The model under review builds one solid part; all positions refer to its coordinate system, in mm. Face numbers are marked on the shaded views. A direction names the side the tool comes from. Give positions to 0.01 mm unless a question says otherwise; leave off trailing zeros. Write each loop counter-clockwise with the first axis right and the second up, starting at its lowest first coordinate (ties: lowest second). Pieces come first, ordered by that corner, then holes. Notation, with made-up numbers: (9.5, 64) -> (44.5, 64) arc R4 ccw to (44.5, 71) -> close; hole circle Ø7 at (-1.5, -3.75). An arc over 180 degrees is marked (long way). Use CSV: the item, a comma, the result in double quotes.
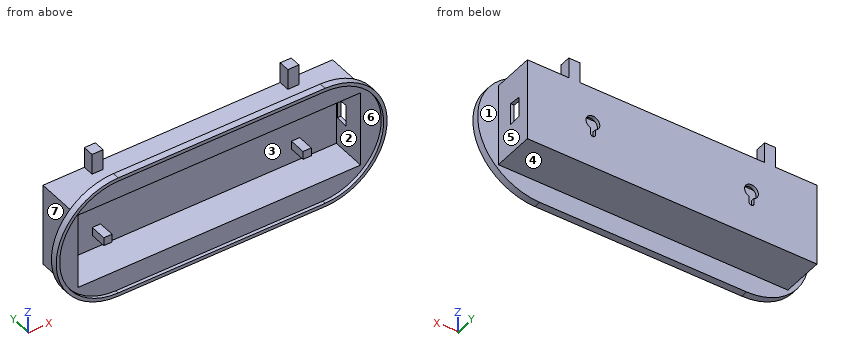
```python
from build123d import *

# Parameters (mm, degrees)
F0_W      = 266.7
F0_H      = 76.2
F1_DEPTH  = 3.175
F2_W      = 266.7
F2_H      = 76.2
F2_W_2    = 260.35
F2_H_2    = 69.85
F3_DEPTH  = 28.956
F4_W      = 260.35
F4_H      = 69.85
F5_DEPTH  = 6.35
F7_DEPTH  = 3.175
F8_W      = 266.7
F8_H      = 76.2
F8_W_2    = 19.05
F8_H_2    = 25.4
F9_DEPTH  = 6.35
F10_W     = 19.05
F10_H     = 25.4
F11_DEPTH = 3.175
F13_DEPTH = 3.175
F14_W     = 10.16
F14_H     = 10.16
F15_DEPTH = 19.05
F16_W     = 7.62
F16_H     = 7.62
F17_DEPTH = 15.24


with BuildPart() as f1:
    # F0 (on Front) → F1 (new body)
    with BuildSketch(Plane.XZ):
        with Locations((133.35, -38.1)):
            Rectangle(F0_W, F0_H)
    extrude(amount=F1_DEPTH)

    # F2 (on face) → F3 (join)
    with BuildSketch(Plane.XZ.offset(3.175)):
        with Locations((133.35, -38.1)):
            Rectangle(F2_W, F2_H)
        with Locations((133.35, -38.1)):
            Rectangle(F2_W_2, F2_H_2, mode=Mode.SUBTRACT)
    extrude(amount=F3_DEPTH)

    # F4 (on face) → F5 (join)
    with BuildSketch(Plane.XZ.offset(32.131)):
        with BuildLine():
            Line((228.6, 19.05), (38.1, 19.05))
            ThreePointArc((38.1, 19.05), (-19.05, -38.1), (38.1, -95.25))
            Line((38.1, -95.25), (228.6, -95.25))
            ThreePointArc((228.6, -95.25), (285.75, -38.1), (228.6, 19.05))
        make_face()
        with Locations((133.35, -38.1)):
            Rectangle(F4_W, F4_H, mode=Mode.SUBTRACT)
    extrude(amount=F5_DEPTH)

    # F6 (on face) → F7 (cut)
    with BuildSketch(Plane.XZ.offset(38.481)):
        with BuildLine():
            Line((228.6, 15.875), (38.1, 15.875))
            ThreePointArc((38.1, 15.875), (-15.875, -38.1), (38.1, -92.075))
            Line((38.1, -92.075), (228.6, -92.075))
            ThreePointArc((228.6, -92.075), (282.575, -38.1), (228.6, 15.875))
        make_face()
    extrude(amount=-F7_DEPTH, mode=Mode.SUBTRACT)

    # F8 (on face) → F9 (join)
    with BuildSketch(Plane(origin=(0, 0, 0), x_dir=(-1, 0, 0), z_dir=(0, 1, 0))):
        with Locations((-133.35, -38.1)):
            Rectangle(F8_W, F8_H)
        with Locations((-206.375, -38.1)):
            Rectangle(F8_W_2, F8_H_2, mode=Mode.SUBTRACT)
        with Locations((-60.325, -38.1)):
            Rectangle(F8_W_2, F8_H_2, mode=Mode.SUBTRACT)
    extrude(amount=F9_DEPTH)

    # F10 (on face) → F11 (join)
    with BuildSketch(Plane(origin=(0, 6.35, 0), x_dir=(-1, 0, 0), z_dir=(0, 1, 0))):
        with Locations((-60.325, -38.1)):
            Rectangle(F10_W, F10_H)
        with BuildLine():
            ThreePointArc((-62.611, -39.198247), (-60.325, -26.924), (-58.039, -39.198247))
            Line((-58.039, -39.198247), (-58.039, -44.45))
            ThreePointArc((-58.039, -44.45), (-60.325, -46.736), (-62.611, -44.45))
            Line((-62.611, -44.45), (-62.611, -39.198247))
        make_face(mode=Mode.SUBTRACT)
        with Locations((-206.375, -38.1)):
            Rectangle(F10_W, F10_H)
        with BuildLine():
            ThreePointArc((-208.661, -39.198247), (-206.375, -26.924), (-204.089, -39.198247))
            Line((-204.089, -39.198247), (-204.089, -44.45))
            ThreePointArc((-204.089, -44.45), (-206.375, -46.736), (-208.661, -44.45))
            Line((-208.661, -44.45), (-208.661, -39.198247))
        make_face(mode=Mode.SUBTRACT)
    extrude(amount=-F11_DEPTH)

    # F12 (on face) → F13 (cut, through all)
    with BuildSketch(Plane.YZ.offset(266.7)):
        Polygon((-4.699, -47.3075), (-4.699, -28.8925), (-15.875, -27.94), (-15.875, -48.26), align=None)
    extrude(amount=-F13_DEPTH, mode=Mode.SUBTRACT)

    # F14 (on face) → F15 (join, through all)
    with BuildSketch(Plane.XY):
        with Locations((43.18, 1.27)):
            Rectangle(F14_W, F14_H)
        with Locations((223.52, 1.27)):
            Rectangle(F14_W, F14_H)
    extrude(amount=F15_DEPTH)

    # F16 (on face) → F17 (join)
    with BuildSketch(Plane.XZ.offset(3.175)):
        with Locations((226.0092, -56.007)):
            Rectangle(F16_W, F16_H)
        with Locations((226.0092, -13.843)):
            Rectangle(F16_W, F16_H)
        with Locations((42.545, -56.007)):
            Rectangle(F16_W, F16_H)
        with Locations((42.545, -13.843)):
            Rectangle(F16_W, F16_H)
    extrude(amount=F17_DEPTH)


solid = f1.part
```
Q1. Consider section C-C (x = 123). Write out the cut boundary in (y, z) (3 decimals), then the cut area to 3 significant figures.
Derived:
outline,"(-38.481, -95.25) -> (-32.131, -95.25) -> (-32.131, -76.2) -> (6.35, -76.2) -> (6.35, 0) -> (-32.131, 0) -> (-32.131, 19.05) -> (-38.481, 19.05) -> (-38.481, 15.875) -> (-35.306, 15.875) -> (-35.306, -3.175) -> (-3.175, -3.175) -> (-3.175, -73.025) -> (-35.306, -73.025) -> (-35.306, -92.075) -> (-38.481, -92.075) -> close"
area,"1,070 mm2"
Q2. Consider section B-B (z = 12). Write out the cut boundary in (x, y), then the cut area to 3 significant figures.
Derived:
outline,"(10.6, -38.48) -> (18.02, -38.48) -> (18.02, -35.31) -> (248.68, -35.31) -> (248.68, -38.48) -> (256.1, -38.48) -> (256.1, -32.13) -> (10.6, -32.13) -> close; (38.1, -3.81) -> (48.26, -3.81) -> (48.26, 6.35) -> (38.1, 6.35) -> close; (218.44, -3.81) -> (228.6, -3.81) -> (228.6, 6.35) -> (218.44, 6.35) -> close"
area,"1,030 mm2"
Q3. Consider section D-D (z = -81.5). Write out the cut boundary in (x, y), then the cut area to 3 significant figures.
Derived:
outline,"(0.92, -38.48) -> (6.01, -38.48) -> (6.01, -35.31) -> (260.69, -35.31) -> (260.69, -38.48) -> (265.78, -38.48) -> (265.78, -32.13) -> (0.92, -32.13) -> close"
area,"873 mm2"
Q4. Machinability: for the marked faces 5, 6 and 7, which of the approach directions +Z, -Z, +X, -X, +Y, -Y give a long, thin tool a straight path to every point of the face, cutting with its end or side? Answer none if there is none.
Derived:
face 5,"+Z, -Z, +X, +Y"
face 6,"-Y"
face 7,"+Z, -Z, -X, +Y"
Q5. Consider section A-A (y = -28). Write out the cut boundary in (x, z) (3 decimals), then the cut area to 3 significant figures.
Derived:
outline,"(0, -76.2) -> (266.7, -76.2) -> (266.7, 0) -> (0, 0) -> close; hole (3.175, -73.025) -> (263.525, -73.025) -> (263.525, -3.175) -> (3.175, -3.175) -> close"
area,"2,140 mm2"
Q6. The part is to be moulded in two halves that separate along Z. For the marked faces 1, 2, 3 and 4, say which applies: pulls with the +Z half, pulls with the -Z half, needs draft (parallel to the pull), parting line crosses it, or undercut.
Derived:
face 1,"needs draft"
face 2,"undercut"
face 3,"undercut"
face 4,"pulls with the -Z half"
Q7. To check wall thickness, follow probe 1 along Z at (x, y) = (104, -19) (3 decimals); probe 2 along X at (y, z) = (-23.5, -39.5) (3 decimals); probe 3 along Y at (x, z) = (73, -88.5). State the ranges of each line that lie inside material, in increasing order.
Derived:
probe 1,"z = -76.2 to -73.025, -3.175 to 0"
probe 2,"x = 0 to 3.175, 263.525 to 266.7"
probe 3,"y = -35.31 to -32.13"
Q8. Insertion check: pin 1 (1.6 mm diameter, centred on x = 207, y = 1.5, fed in from -Z); pin 2 (9.5 mm diameter, centred on x = 207, z = -39.5, fed in from -Y) (3 decimals); pin 3 (1.6 mm diameter, centred on y = 4, z = -43, fed in from -X). Each pin has a flat end and moves straight along its axis. Give the tip position at first contact, or say it passes through.
Derived:
pin 1,"stops at z = -76.2"
pin 2,"stops at y = -3.175"
pin 3,"stops at x = 0"
